Geometry: final body of the model. Coordinates: model frame, mm. Face numbers are marked on the shaded views. A direction names the side the tool comes from. Give positions to 0.01 mm unless a question says otherwise; leave off trailing zeros. Loops run counter-clockwise (first coordinate to the right, second up) from the corner with the lowest first, then second, coordinate; pieces in that order, holes last. Notation, with made-up numbers: (21, 20.25) - (41, 20.25) arc R22 cw to (41, 31.25) - close; hole circle Ø6 at (17, -31). An arc over 180 degrees is marked (long way). Use CSV: the item, a comma, the result in double quotes. Start each with the question number.
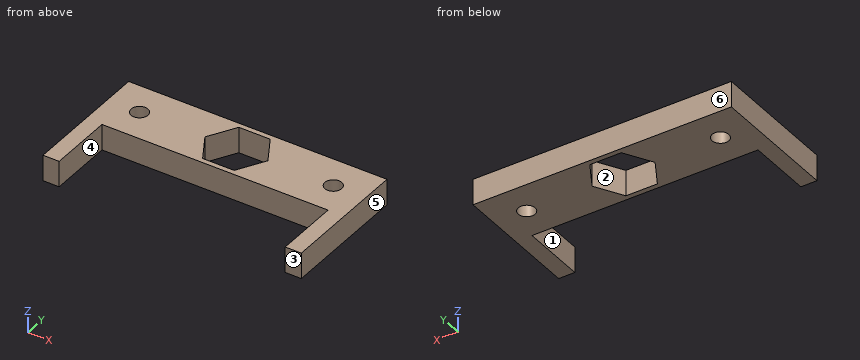
Autodesk Inventor part; units mm, degrees
ref_plane "YZ Plane" through (0, 0, 0) normal (1, 0, 0) x (0, 1, 0)
ref_plane "XZ Plane" through (0, 0, 0) normal (0, 1, 0) x (-1, 0, 0)
ref_plane "XY Plane" through (0, 0, 0) normal (0, 0, 1) x (1, 0, 0)
sketch "Sketch1" plane through (0, 0, 0) normal (0, 0, 1) x (1, 0, 0)
  line L0 (40, -10) -> (-40, -10)
  line L1 (-40, -10) -> (-40, 10)
  line L2 (-40, 10) -> (40, 10)
  line L3 (40, 10) -> (40, -10)
  line L4 (0, -14) -> (0, 14)
  line L5 (40, -10) -> (30, -10)
  line L6 (-56, 0) -> (56, 0)
  circle A0 centre (-0.5449, 0.9437) radius 3.3235
  line L7 (-4.875, -6.5563) -> (-9.2051, 0.9437)
  line L8 (-9.2051, 0.9437) -> (-4.875, 8.4437)
  line L9 (-4.875, 8.4437) -> (3.7853, 8.4437)
  line L10 (3.7853, 8.4437) -> (8.1154, 0.9437)
  line L11 (8.1154, 0.9437) -> (3.7853, -6.5563)
  line L12 (3.7853, -6.5563) -> (-4.875, -6.5563)
  circle A1 centre (-0.5449, 0.9437) radius 3.3235
  line L13 (-4.875, -6.5563) -> (-9.2051, 0.9437)
  line L14 (-9.2051, 0.9437) -> (-4.875, 8.4437)
  line L15 (-4.875, 8.4437) -> (3.7853, 8.4437)
  line L16 (3.7853, 8.4437) -> (8.1154, 0.9437)
  line L17 (8.1154, 0.9437) -> (3.7853, -6.5563)
  line L18 (3.7853, -6.5563) -> (-4.875, -6.5563)
  point P0 (0, 0)
  dimension "d0" = 80
  dimension "d1" = 20
  dimension "d70" = 40
  dimension "d73" = 10
extrude "Extrusion1" add sketch "Sketch1" against normal blind 8
sketch "Sketch3" plane through (0, 0, 0) normal (0, 0, 1) x (1, 0, 0)
  line L0 (0, -14) -> (0, 14)
  line L1 (-56, 0) -> (56, 0)
  line L2 (-4.875, 8.4437) -> (4.875, 8.4437)
  line L3 (4.875, 8.4437) -> (9.75, 0)
  line L4 (9.75, 0) -> (4.875, -8.4437)
  line L5 (4.875, -8.4437) -> (-4.875, -8.4437)
  line L6 (-4.875, -8.4437) -> (-9.75, 0)
  line L7 (-9.75, 0) -> (-4.875, 8.4437)
  point P0 (0, 0)
  point P1 (0, 0)
  dimension "d65" = 19.5
extrude "Extrusion2" cut sketch "Sketch3" against normal blind 10
sketch "Sketch9" plane through (0, 0, -8) normal (0, 0, -1) x (-1, 0, 0)
  circle A0 centre (-30, 0) radius 2.6
  line L0 (0, -14) -> (0, 14)
  line L1 (56, 0) -> (-56, 0)
  circle A1 centre (30, 0) radius 2.6
  dimension "d40" = 5.2
  dimension "d41" = 60
extrude "Extrusion3" cut sketch "Sketch9" against normal through all
sketch "Sketch14" plane through (0, 0, 0) normal (0, 0, 1) x (1, 0, 0)
  circle A0 centre (30, 0) radius 2.6
  circle A1 centre (-30, 0) radius 2.6
  line L0 (-9.75, 0) -> (-4.875, 8.4437)
  line L1 (-4.875, 8.4437) -> (4.875, 8.4437)
  line L2 (4.875, 8.4437) -> (9.75, 0)
  line L3 (9.75, 0) -> (4.875, -8.4437)
  line L4 (4.875, -8.4437) -> (-4.875, -8.4437)
  line L5 (-4.875, -8.4437) -> (-9.75, 0)
  line L6 (40, -10) -> (-40, -10)
  line L7 (40, 10) -> (40, -10)
  line L8 (-40, 10) -> (40, 10)
  line L9 (-40, -10) -> (-40, 10)
  line L10 (-40, -10) -> (-35, -10)
  line L11 (-35, -10) -> (-35, -30)
  line L12 (-35, -30) -> (-40, -30)
  line L13 (-40, -30) -> (-40, -10)
  line L14 (-56, 0) -> (56, 0)
  line L15 (0, -33.313) -> (0, 17.2188)
  line L16 (40, -10) -> (35, -10)
  line L17 (35, -10) -> (35, -30)
  line L18 (35, -30) -> (40, -30)
  line L19 (40, -30) -> (40, -10)
  point P0 (0, 0)
  dimension "d74" = 5
  dimension "d75" = 20
extrude "Extrusion7" add sketch "Sketch14" against normal blind 8 contours L19 L18 L17 L6 | L11 L12 L13 L6
properties part number "drive_support" material "ABS Plastic"
Item 1: Mould query, pull axis X, two halves, no side actions, for the marked faces 4, 5 and 6. Classes: pulls with the +X half, pulls with the -X half, needs draft (parallel to the pull), parting line crosses it, or undercut.
Item 2: Pin query (flat end, axial travel): pin 1 Ø4 at (x, z) = (2.5, -4.5) entering from -Y. Return the tip coordinate at first contact, or that it passes through.
Item 3: Section A-A (z = -5.25). Output: boundary loops of the cut face in (x, y) (3 decimals), plus the area to 3 significant figures.
Item 4: Reachability of the marked faces 1, 2 and 3 from +Z, -Z, +X, -X, +Y, -Y: full face, straight path, thin tool, end or side. Return the list, or none.
Item 5: Section C-C (y = -17). Output: boundary loops of the cut face in (x, z), plus the area to 3 significant figures.
Item 6: Section B-B (x = -30). Output: boundary loops of the cut face in (y, z).
Item 7: Ray query, probe 1 along X at (y, z) = (0, -5); probe 2 along Y at (x, z) = (30, -5.75); probe 3 along Y at (x, z) = (-3, -2.25). Return the intervals inside material, ascending.
Item 8: Section D-D (x = -14). Output: boundary loops of the cut face in (y, z), plus the area to 3 significant figures.
Outcome:
1,face 4,"undercut"
1,face 5,"pulls with the +X half"
1,face 6,"needs draft"
2,pin 1,"stops at y = -10"
3,outline,"(-40, -30) - (-35, -30) - (-35, -10) - (35, -10) - (35, -30) - (40, -30) - (40, 10) - (-40, 10) - close; hole circle Ø5.2 at (-30, 0); hole (-9.75, 0) - (-4.875, -8.444) - (4.875, -8.444) - (9.75, 0) - (4.875, 8.444) - (-4.875, 8.444) - close; hole circle Ø5.2 at (30, 0)"
3,area,"1,510 mm2"
4,face 1,"+Z, -Z, -Y"
4,face 2,"+Z, -Z"
4,face 3,"+Z, -Z, +X, -X, -Y"
5,outline,"(-40, -8) - (-35, -8) - (-35, 0) - (-40, 0) - close; (35, -8) - (40, -8) - (40, 0) - (35, 0) - close"
5,area,"80.0 mm2"
6,outline,"(-10, -8) - (-2.6, -8) - (-2.6, 0) - (-10, 0) - close; (2.6, -8) - (10, -8) - (10, 0) - (2.6, 0) - close"
7,probe 1,"x = -40 to -32.6, -27.4 to -9.75, 9.75 to 27.4, 32.6 to 40"
7,probe 2,"y = -10 to -2.6, 2.6 to 10"
7,probe 3,"y = -10 to -8.44, 8.44 to 10"
8,outline,"(-10, -8) - (10, -8) - (10, 0) - (-10, 0) - close"
8,area,"160 mm2"
